```python
from build123d import *

# Parameters (mm, degrees)
SKETCH3_W           = 25.4
SKETCH3_H           = 25.4
SKETCH3_W_2         = 19.304
SKETCH3_H_2         = 19.304
BOSS_EXTRUDE1_DEPTH = 2830
FILLET1_R           = 2.5
FILLET2_R           = 1


with BuildPart() as part:
    # Sketch3 → Boss-Extrude1 (new body)
    with BuildSketch(Plane(origin=(0, 0, 0), x_dir=(0, 0, -1), z_dir=(1, 0, 0))):
        Rectangle(SKETCH3_W, SKETCH3_H)
        Rectangle(SKETCH3_W_2, SKETCH3_H_2, mode=Mode.SUBTRACT)
    extrude(amount=-BOSS_EXTRUDE1_DEPTH)

    # Fillet1
    fillet1_edges = [part.edges().sort_by_distance(p)[0] for p in [
        (-1415, -12.7, -12.7),
        (-1415, -12.7, 12.7),
        (-1415, 12.7, 12.7),
        (-1415, 12.7, -12.7),
    ]]
    fillet(fillet1_edges, radius=FILLET1_R)

    # Fillet2
    fillet2_edges = [part.edges().sort_by_distance(p)[0] for p in [
        (-1415, 9.652, -9.652),
        (-1415, -9.652, -9.652),
        (-1415, -9.652, 9.652),
        (-1415, 9.652, 9.652),
    ]]
    fillet(fillet2_edges, radius=FILLET2_R)


solid = part.part
```
Part model, mm, in its own coordinate system. Round coordinates to 2 decimals unless told otherwise and drop trailing zeros. Loops run counter-clockwise (first coordinate to the right, second up) from the corner with the lowest first, then second, coordinate; pieces in that order, holes last. Notation, with made-up numbers: (17.5, 21.25) -> (32.5, 21.25) arc R20 cw to (32.5, 46.25) -> close; hole circle Ø6 at (0.25, 12). An arc over 180 degrees is marked (long way). Use CSV: the item, a comma, the result in double quotes. Start each with the question number.
1) Wall check: L1, parallel to Z at x = -1983, y = 3.25; L2, parallel to Y at x = -1625.5, z = -11.5. Give the ranges that are in metal, low to high. Write a range as [from, to].
2) Drop a flat-ended pin along its axis: P1, Ø8, axis at y = 4.5, z = 1.5, coming from the +X side. Give the stop position or say it passes through.
3) Cut at C-C, the plane x = -2196. Write the cut outline in (y, z), plus the area to 3 significant figures.
4) Cut at A-A, the plane y = -0.75. Write the cut outline in (x, z), plus the area to 3 significant figures.
Determined:
1,L1,"z = [-12.7, -9.65], [9.65, 12.7]"
1,L2,"y = [-12.34, 12.34]"
2,P1,"passes through"
3,outline,"(-12.7, -10.2) arc R2.5 ccw to (-10.2, -12.7) -> (10.2, -12.7) arc R2.5 ccw to (12.7, -10.2) -> (12.7, 10.2) arc R2.5 ccw to (10.2, 12.7) -> (-10.2, 12.7) arc R2.5 ccw to (-12.7, 10.2) -> close; hole (-9.65, -8.65) arc R1 ccw to (-8.65, -9.65) -> (8.65, -9.65) arc R1 ccw to (9.65, -8.65) -> (9.65, 8.65) arc R1 ccw to (8.65, 9.65) -> (-8.65, 9.65) arc R1 ccw to (-9.65, 8.65) -> close"
3,area,"268 mm2"
4,outline,"(-2830, -12.7) -> (0, -12.7) -> (0, -9.65) -> (-2830, -9.65) -> close; (-2830, 9.65) -> (0, 9.65) -> (0, 12.7) -> (-2830, 12.7) -> close"
4,area,"17,300 mm2"
